Autodesk Inventor part; units mm, degrees
ref_plane "YZ Plane" through (0, 0, 0) normal (1, 0, 0) x (0, 1, 0)
ref_plane "XZ Plane" through (0, 0, 0) normal (0, 1, 0) x (-1, 0, 0)
ref_plane "XY Plane" through (0, 0, 0) normal (0, 0, 1) x (1, 0, 0)
sketch "草圖1" plane through (0, 0, 0) normal (0, 0, 1) x (1, 0, 0)
  line L0 (30, -250) -> (-30, -250)
  line L1 (-30, -250) -> (-30, 250)
  line L2 (-30, 250) -> (30, 250)
  line L3 (30, 250) -> (30, -250)
  line L4 (30, -250) -> (-30, 250) construction
  line L5 (-30, -250) -> (30, 250) construction
  point P0 (0, 0)
  dimension "d0" = 60
  dimension "d1" = 500
extrude "擠出1" add sketch "草圖1" along normal blind 30
sketch "草圖2" plane through (30, -250, 0) normal (1, 0, 0) x (0, 0, -1)
  line L0 (0, 500) -> (0, 0)
  line L1 (0, 0) -> (-42.4264, -42.4264)
  line L2 (0, 0) -> (60, 0) construction
  line L3 (-42.4264, -42.4264) -> (-42.4264, -22.4264)
  line L4 (-42.4264, -22.4264) -> (-62.4264, -22.4264)
  line L5 (-62.4264, -22.4264) -> (-23.4773, 16.5227)
  line L6 (0, 0) -> (-23.4773, 16.5227)
  line L7 (0, 500) -> (-42.4264, 542.4264)
  line L8 (-42.4264, 542.4264) -> (-42.4264, 522.4264)
  line L9 (-42.4264, 522.4264) -> (-62.4264, 522.4264)
  line L10 (-62.4264, 522.4264) -> (-16.5227, 476.5227)
  line L11 (-16.5227, 476.5227) -> (0, 500)
  point P0 (0, 250)
  dimension "d4" = 60
  dimension "d5" = 135
  dimension "d6" = 20
  dimension "d7" = 20
  dimension "d8" = 60
  dimension "d9" = 20
  dimension "d10" = 20
extrude "擠出2" add sketch "草圖2" against normal blind 60
properties part number "DOF5"
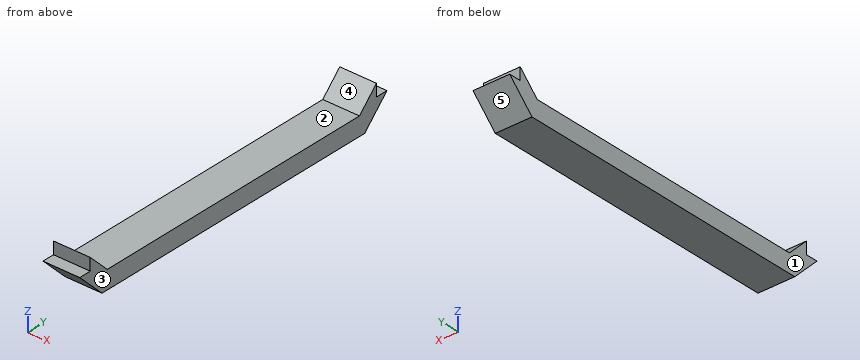
Geometry check sheet. Reference: the model listing, model coordinates, mm. Face numbers are marked on the shaded views. A direction names the side the tool comes from. Round coordinates to 2 decimals unless told otherwise and drop trailing zeros. Write each loop counter-clockwise with the first axis right and the second up, starting at its lowest first coordinate (ties: lowest second). Pieces come first, ordered by that corner, then holes. Notation, with made-up numbers: (-32.5, 24.25) -> (6.5, 24.25) arc R23 ccw to (6.5, 39.25) -> close; hole circle Ø6 at (6, 76.25). An arc over 180 degrees is marked (long way). One line per item, written item: value. Start each with the question number.
(1) Access from +Z, -Z, +X, -X, +Y, -Y to the whole of each face (thin tool, end or side, straight path). Record for the marked faces 1 and 2.
(2) Draft check along Y on the marked faces 3, 4 and 5. Enter one of: +Y half, -Y half, draft (parallel to the pull), parting line (faces both ways), or undercut.
(3) Scan lines: line 1 (Z direction, x = 6.5, y = -58); line 2 (Y direction, x = 19, z = 45); line 3 (Y direction, x = -6, z = 32). Record each from-to range of solid material in increasing order. Write a range as [from, to].
(4) Cross-section at A-A, the plane z = 56. Record the cut outline in (x, y), and give its area (3 significant figures).
(5) Cross-section at C-C, the plane z = 19. Record the cut outline in (x, y).
(6) Go/stop test with flat-tipped pins: pin 1 Ø5 at (x, y) = (-10, -194) entering from +Z; pin 2 Ø12 at (x, z) = (-15.5, 31) entering from +Y; pin 3 Ø6 at (x, y) = (17, 232.5) entering from -Z; pin 4 Ø6 at (x, z) = (-21, 19.5) entering from -Y. Record where each tip stops, or that it passes through.
(7) Cross-section at D-D, the plane y = -58. Record the cut outline in (x, z), and give its area (3 significant figures).
(8) Cross-section at B-B, the plane x = 17. Record the cut outline in (y, z).
Answer:
1. face 1: +Z, -Z, -X, +Y, -Y
1. face 2: +Z, +X, -X
2. face 3: draft
2. face 4: undercut
2. face 5: +Y half
3. line 1: [0, 30]
3. line 2: [-272.43, -255], [255, 272.43]
3. line 3: [-282, -242], [242, 282]
4. outline: (-30, -272.43) -> (30, -272.43) -> (30, -266) -> (-30, -266) -> close; (-30, 266) -> (30, 266) -> (30, 272.43) -> (-30, 272.43) -> close
4. area: 771 mm²
5. outline: (-30, -269) -> (30, -269) -> (30, 269) -> (-30, 269) -> close
6. pin 1: z = 30
6. pin 2: y = 287
6. pin 3: z = 0
6. pin 4: y = -272.5
7. outline: (-30, 0) -> (30, 0) -> (30, 30) -> (-30, 30) -> close
7. area: 1,800 mm²
8. outline: (-292.43, 42.43) -> (-250, 0) -> (250, 0) -> (292.43, 42.43) -> (272.43, 42.43) -> (272.43, 62.43) -> (240, 30) -> (-240, 30) -> (-272.43, 62.43) -> (-272.43, 42.43) -> close
